Could you check a few things on this model? Use its own coordinates, in mm. A direction names the side the tool comes from. Coordinates: 2 decimals unless noted, no trailing zeros. Write each loop counter-clockwise with the first axis right and the second up, starting at its lowest first coordinate (ties: lowest second). Pieces come first, ordered by that corner, then holes. Notation, with made-up numbers: (3.25, -7.75) - (61.25, -7.75) arc R16 cw to (61.25, 3.25) - close; hole circle Ø10 at (72, 20.25). An arc over 180 degrees is marked (long way). Answer as a JSON object with one key per item and string values. Group by question number.
1) If we section it at C-C (z = 34): Write out the boundary of the cut face in (x, y), plus the area to 3 significant figures.
2) If we section it at B-B (y = -3): Write out the boundary of the cut face in (x, z).
3) If we section it at D-D (z = 28.5): Write out the boundary of the cut face in (x, y).
4) Will this pin go through, and if not, where does the flat tip stop? pin 1 Ø3 at (y, z) = (1, 3) entering from +X.
5) If we section it at A-A (x = 0): Write out the boundary of the cut face in (y, z).
6) On a 3-axis mill with a long thin cutter (end or side, diameter ignored), from which of +Z, -Z, +X, -X, +Y, -Y can I reach the whole of each face in a straight line? I mean faces 4 (the flat face through (-4, 0, 20)), 5 (the flat face through (-5, 0, 20)). Say none if no direction works.
7) Please list where these lines run through material, in increasing order: line 1 along Y through (x, z) = (3.5, 38.5); line 2 along Y through (x, z) = (-4.25, 3).
8) We'd pull the mould along Z, two halves only. Please class faces 1 (the cylindrical face through (4.507, -0.952, 3.434)), 2 (the flat face through (-4.5, 0.1, 40)), 3 (the flat face through (0, -4, 20)): released by +Z, released by -Z, zero draft, split by the parting line, or undercut.
```python
from build123d import *

# Parameters (mm, degrees)
SKIZZE1_W                       = 10
SKIZZE1_H                       = 10
SKIZZE1_W_2                     = 8
SKIZZE1_H_2                     = 8
AUFSATZ_LINEAR_AUSTRAGEN1_DEPTH = 40
SKIZZE2_R                       = 2
SCHNITT_LINEAR_AUSTRAGEN1_DEPTH = 42.533119315
SKIZZE3_R                       = 2.5
SCHNITT_LINEAR_AUSTRAGEN2_DEPTH = 17


with BuildPart() as part:
    # Skizze1 → Aufsatz-Linear austragen1 (new body)
    with BuildSketch(Plane.XY):
        Rectangle(SKIZZE1_W, SKIZZE1_H)
        Rectangle(SKIZZE1_W_2, SKIZZE1_H_2, mode=Mode.SUBTRACT)
    extrude(amount=AUFSATZ_LINEAR_AUSTRAGEN1_DEPTH)

    # Skizze2 → Schnitt-Linear austragen1 (cut, through all)
    with BuildSketch(Plane(origin=(5, 0, 0), x_dir=(0, 0, -1), z_dir=(1, 0, 0))):
        with Locations((-34, 1)):
            Circle(SKIZZE2_R)
        with Locations((-3, 1)):
            Circle(SKIZZE2_R)
    extrude(amount=-SCHNITT_LINEAR_AUSTRAGEN1_DEPTH, mode=Mode.SUBTRACT)

    # Skizze3 → Schnitt-Linear austragen2 (cut)
    with BuildSketch(Plane(origin=(0, 5, 0), x_dir=(1, 0, 0), z_dir=(0, 1, 0))):
        with Locations(Location((0, -13, 0), (0, 0, 270))):
            Circle(SKIZZE3_R)
    extrude(amount=-SCHNITT_LINEAR_AUSTRAGEN2_DEPTH, mode=Mode.SUBTRACT)


solid = part.part
```
Here are the results:
{
 "1": {"outline": "(-5, -5) - (5, -5) - (5, -1) - (4, -1) - (4, -4) - (-4, -4) - (-4, -1) - (-5, -1) - close; (-5, 3) - (-4, 3) - (-4, 4) - (4, 4) - (4, 3) - (5, 3) - (5, 5) - (-5, 5) - close", "area": "28.0 mm²"},
 "2": {"outline": "(-5, 0) - (-4, 0) - (-4, 40) - (-5, 40) - close; (4, 0) - (5, 0) - (5, 40) - (4, 40) - close"},
 "3": {"outline": "(-5, -5) - (5, -5) - (5, 5) - (-5, 5) - close; hole (-4, -4) - (4, -4) - (4, 4) - (-4, 4) - close"},
 "4": {"pin 1": "passes through"},
 "5": {"outline": "(-5, 0) - (-4, 0) - (-4, 10.5) - (-5, 10.5) - close; (-5, 15.5) - (-4, 15.5) - (-4, 40) - (-5, 40) - close; (4, 0) - (5, 0) - (5, 10.5) - (4, 10.5) - close; (4, 15.5) - (5, 15.5) - (5, 40) - (4, 40) - close"},
 "6": {"face 4": "+Z, -Z", "face 5": "+Z, -Z, -X, +Y, -Y"},
 "7": {"line 1": "y = -5 to -4, 4 to 5", "line 2": "y = -5 to -1, 3 to 5"},
 "8": {"face 1": "undercut", "face 2": "released by +Z", "face 3": "zero draft"}
}
